from build123d import *

# Parameters (mm, degrees)
SKETCH1_R           = 0.467713673
BOSS_EXTRUDE1_DEPTH = 3


with BuildPart() as part:
    # Sketch1 → Boss-Extrude1 (new body)
    with BuildSketch(Plane.XY):
        with BuildLine():
            Line((-7.145342709, -3), (6.320992929, -3))
            ThreePointArc((6.320992929, -3), (9.320992929, 0), (6.320992929, 3))
            Line((6.320992929, 3), (-7.145342709, 3))
            Line((-7.145342709, 3), (-7.145342709, -3))
        make_face()
        with Locations((6.320992929, 0)):
            Circle(SKETCH1_R, mode=Mode.SUBTRACT)
        with BuildLine():
            Line((-6.001882726, 1.5), (-6.001882726, -1.5))
            ThreePointArc((-6.001882726, -1.5), (-2.679007071, 0), (-6.001882726, 1.5))
        make_face(mode=Mode.SUBTRACT)
    extrude(amount=BOSS_EXTRUDE1_DEPTH)


solid = part.part
Build history of the part. All positions in model axes, mm. A direction names the side the tool comes from. Round coordinates to 2 decimals unless told otherwise and drop trailing zeros. Write each loop counter-clockwise with the first axis right and the second up, starting at its lowest first coordinate (ties: lowest second). Pieces come first, ordered by that corner, then holes. Notation, with made-up numbers: (87, 65) - (104, 65) arc R10 cw to (104, 74) - close; hole circle Ø9 at (82.25, 72). An arc over 180 degrees is marked (long way). One line per question, with ' | ' between items.
1. Band-saw the part on C-C, the plane y = -1.3. Write the cut outline in (x, z).
Results are:
outline: (-7.15, 0) - (-6, 0) - (-6, 3) - (-7.15, 3) - close; (-3.16, 0) - (9.02, 0) - (9.02, 3) - (-3.16, 3) - close
2. Band-saw the part on D-D, the plane y = 2.35. Write the cut outline in (x, z).
Results are:
outline: (-7.15, 0) - (8.19, 0) - (8.19, 3) - (-7.15, 3) - close
3. Mould opens along Y. For faces 1 (the face through (6.767, 0.14, 1.479)), 2 (the face through (1, 0, 3)), 3 (the face through (0, 3, 1)) say: released by +Y, released by -Y, zero draft, split by the parting line, or undercut.
Results are:
face 1: undercut | face 2: zero draft | face 3: released by +Y
4. Band-saw the part on B-B, the plane z = 2.7. Write the cut outline in (x, y).
Results are:
outline: (-7.15, -3) - (6.32, -3) arc R3 ccw to (6.32, 3) - (-7.15, 3) - close; hole (-6, -1.5) arc R2 ccw (long way) to (-6, 1.5) - close; hole circle Ø0.94 at (6.32, 0)
5. Drill centre lines: line 1 along X through (y, z) = (0.25, 2.7); line 2 along Y through (x, z) = (-3.5, 1.1); line 3 along Y through (x, z) = (6.5, 2.6). Where is each one in solid material? Low to high. Write a range as from..to.
Results are:
line 1: -7.15..-6, -2.69..5.93, 6.72..9.31 | line 2: -3..-1.62, 1.62..3 | line 3: -2.99..-0.43, 0.43..2.99
6. Band-saw the part on A-A, the plane y = 0. Write the cut outline in (x, z).
Results are:
outline: (-7.15, 0) - (-6, 0) - (-6, 3) - (-7.15, 3) - close; (-2.68, 0) - (5.85, 0) - (5.85, 3) - (-2.68, 3) - close; (6.79, 0) - (9.32, 0) - (9.32, 3) - (6.79, 3) - close
7. Tool access for faces 4 (the face through (-6.002, 0, 1)), 5 (the face through (9.32, -0.07, 1.48)): list every direction of +Z, -Z, +X, -X, +Y, -Y with a clear straight run to the whole face (end or side of a thin tool).
Results are:
face 4: +Z, -Z | face 5: +Z, -Z, +X
